The listing builds one solid part. Answer for the finished solid, in the listing's coordinates (mm). A direction names the side the tool comes from. Give positions to 0.01 mm unless a question says otherwise; leave off trailing zeros. Order: outer loops, then holes, each group sorted by start corner. A loop starts at its lowest first (then second) coordinate and runs counter-clockwise, first axis right, second up. Notation, with made-up numbers: (69.25, 3.25) - (125.25, 3.25) arc R28 ccw to (125.25, 38.25) - close; hole circle Ø8 at (83, -20.5). An arc over 180 degrees is marked (long way). Use CSV: the item, a comma, the result in double quotes.
Autodesk Inventor part; units mm, degrees
ref_plane "YZ Plane" through (0, 0, 0) normal (1, 0, 0) x (0, 1, 0)
ref_plane "XZ Plane" through (0, 0, 0) normal (0, 1, 0) x (-1, 0, 0)
ref_plane "XY Plane" through (0, 0, 0) normal (0, 0, 1) x (1, 0, 0)
sketch "Sketch1" plane through (0, 0, 0) normal (0, 0, 1) x (1, 0, 0)
  arc A0 (18.1843, -16.5324) -> (18.7618, -13.101) centre (16.0629, -14.4111) ccw
  arc A1 (18.7618, 13.101) -> (18.7618, -13.101) centre (45.75, 0) ccw
  arc A2 (18.7618, 13.101) -> (18.1843, 16.5324) centre (16.0629, 14.4111) ccw
  line L0 (11.5324, 23.1843) -> (18.1843, 16.5324)
  arc A3 (11.5324, 23.1843) -> (8.101, 23.7618) centre (9.4111, 21.0629) ccw
  arc A4 (-18.101, 23.7618) -> (8.101, 23.7618) centre (-5, 50.75) ccw
  arc A5 (-18.101, 23.7618) -> (-21.5324, 23.1843) centre (-19.4111, 21.0629) ccw
  line L1 (-28.1843, 16.5324) -> (-21.5324, 23.1843)
  arc A6 (-28.1843, 16.5324) -> (-28.7618, 13.101) centre (-26.0629, 14.4111) ccw
  arc A7 (-28.7618, -13.101) -> (-28.7618, 13.101) centre (-55.75, 0) ccw
  arc A8 (-28.7618, -13.101) -> (-28.1843, -16.5324) centre (-26.0629, -14.4111) ccw
  line L2 (-21.5324, -23.1843) -> (-28.1843, -16.5324)
  arc A9 (-21.5324, -23.1843) -> (-18.101, -23.7618) centre (-19.4111, -21.0629) ccw
  arc A10 (8.101, -23.7618) -> (-18.101, -23.7618) centre (-5, -50.75) ccw
  arc A11 (8.101, -23.7618) -> (11.5324, -23.1843) centre (9.4111, -21.0629) ccw
  line L3 (18.1843, -16.5324) -> (11.5324, -23.1843)
  circle A12 centre (10, -15) radius 4
  circle A13 centre (-20, -15) radius 4
  circle A14 centre (-20, 15) radius 4
  circle A15 centre (10, 15) radius 4
  circle A16 centre (-5, 0) radius 13
  line L4 (39.4645, -4.5) -> (34.9645, -4.5)
  line L5 (34.9645, -4.5) -> (34.9645, 4.5)
  line L6 (34.9645, 4.5) -> (39.4645, 4.5)
  line L7 (39.4645, 4.5) -> (39.4645, 10)
  line L8 (39.4645, 10) -> (31.4645, 10)
  line L9 (31.4645, 10) -> (31.4645, -10)
  line L10 (31.4645, -10) -> (39.4645, -10)
  line L11 (39.4645, -10) -> (39.4645, -4.5)
  line L12 (31.4645, -10) -> (31.4645, -17.0711)
  line L13 (31.4645, -17.0711) -> (24.4726, -24.0629)
  line L14 (31.4645, 10) -> (31.4645, 17.0711)
  line L15 (-19.4111, -24.0629) -> (24.4726, -24.0629)
  line L16 (-19.4111, 24.0629) -> (24.4726, 24.0629)
  line L17 (31.4645, 17.0711) -> (24.4726, 24.0629)
  circle A17 centre (-78.5, 0) radius 12.5
  line L18 (-19.9788, -24.0087) -> (-80.8656, -12.2741)
  line L19 (-80.8656, 12.2741) -> (-19.9788, 24.0087)
  point P0 (0, 0)
  dimension "d0" = 45
  dimension "d1" = 5
  dimension "d4" = 78.5
  dimension "d5" = 25
extrude "Extrusion1" add sketch "Sketch1" along normal blind 10 contours L3 A11 A10 A9 L2 A8 A7 A6 L1 A5 A4 A3 L0 A2 A1 A0 | A0 A1 A2 L0 A3 L16 L17 L14 L9 L12 L13 L15 A11 L3 | L15 A9 A10 A11 | L18 A17 L19 A5 L1 A6 A7 A8 L2 A9 | A3 A4 A5 L16 | A17
sketch "Sketch2" plane through (0, 0, 0) normal (0, 0, -1) x (-1, 0, 0)
  line L0 (-24.4726, -24.0629) -> (-31.4645, -17.0711)
  line L1 (19.4111, -24.0629) -> (-24.4726, -24.0629)
  arc A0 (19.4111, -24.0629) -> (19.9788, -24.0087) centre (19.4111, -21.0629) ccw
  line L2 (80.8656, -12.2741) -> (19.9788, -24.0087)
  arc A1 (80.8656, -12.2741) -> (80.8656, 12.2741) centre (78.5, 0) ccw
  line L3 (19.9788, 24.0087) -> (80.8656, 12.2741)
  arc A2 (19.9788, 24.0087) -> (19.4111, 24.0629) centre (19.4111, 21.0629) ccw
  line L4 (-24.4726, 24.0629) -> (19.4111, 24.0629)
  line L5 (-31.4645, 17.0711) -> (-24.4726, 24.0629)
  line L6 (-31.4645, -17.0711) -> (-31.4645, 17.0711)
  circle A3 centre (-10, -15) radius 4
  circle A4 centre (20, -15) radius 4
  circle A5 centre (20, 15) radius 4
  circle A6 centre (-10, 15) radius 4
  circle A7 centre (5, 0) radius 13
  line L7 (-31.4645, 17.0711) -> (-23.4645, 17.0711)
  line L8 (-23.4645, 17.0711) -> (-23.4645, -17.0711)
  line L9 (-24.4726, -24.0629) -> (-31.4645, -17.0711)
  line L10 (-23.4645, -17.0711) -> (-31.4645, -17.0711)
  line L11 (-23.4645, 17.0711) -> (-19.4726, 21.0629)
  line L12 (-19.4726, 21.0629) -> (-19.4726, 24.0629)
  line L13 (-23.4645, -17.0711) -> (-19.4726, -21.0629)
  line L14 (-19.4726, -21.0629) -> (-19.4726, -24.0629)
  line L15 (19.4111, -24.0629) -> (-24.4726, -24.0629)
  point P0 (0, 0)
  dimension "d6" = 8
  dimension "d9" = 3
extrude "Extrusion2" add sketch "Sketch2" along normal blind 29.9 contours L0 L10 L13 L14 L1 | L6 L7 L8 L10 | L5 L4 L12 L11 L7
sketch "Sketch3" plane through (23.4645, -17.0711, 0) normal (-1, 0, 0) x (0, 0, 1)
  line L0 (0, 34.1421) -> (0, 0)
  line L1 (0, 34.1421) -> (-29.9, 34.1421)
  line L2 (-29.9, 0) -> (-29.9, 34.1421)
  line L3 (0, 0) -> (-29.9, 0)
  point P0 (0, 17.0711)
  point P1 (-1.95, 25.0158)
  point P2 (-17.95, 25.0158)
  point P3 (-17.95, 10.0158)
  point P4 (-1.95, 10.0158)
  dimension "d10" = 15
  dimension "d11" = 16
  dimension "d12" = 11.95
hole "Hole1" at (23.4645, 7.9447, -1.95) at (23.4645, 7.9447, -17.95) at (23.4645, -7.0553, -17.95) at (23.4645, -7.0553, -1.95) direction (1, 0, 0) diameter 3.6 end through all counterbore diameter 6.5 counterbore depth 3.4
sketch "Sketch4" plane through (0, 0, 0) normal (0, 0, -1) x (-1, 0, 0)
  circle A0 centre (5, 0) radius 13
  circle A1 centre (-10, 15) radius 4
  circle A2 centre (20, 15) radius 4
  circle A3 centre (20, -15) radius 4
  circle A4 centre (-10, -15) radius 4
  line L0 (-19.4726, 24.0629) -> (-19.4726, 21.0629)
  line L1 (-19.4726, 21.0629) -> (-23.4645, 17.0711)
  line L2 (-23.4645, 17.0711) -> (-23.4645, 10.5447)
  line L3 (-23.4645, 10.5447) -> (-23.4645, 5.3447)
  line L4 (-23.4645, 5.3447) -> (-23.4645, -4.4553)
  line L5 (-23.4645, -4.4553) -> (-23.4645, -9.6553)
  line L6 (-23.4645, -9.6553) -> (-23.4645, -17.0711)
  line L7 (-23.4645, -17.0711) -> (-19.4726, -21.0629)
  line L8 (-19.4726, -21.0629) -> (-19.4726, -24.0629)
  line L9 (19.4111, -24.0629) -> (-19.4726, -24.0629)
  arc A5 (19.4111, -24.0629) -> (19.9788, -24.0087) centre (19.4111, -21.0629) ccw
  line L10 (80.8656, -12.2741) -> (19.9788, -24.0087)
  arc A6 (80.8656, -12.2741) -> (80.8656, 12.2741) centre (78.5, 0) ccw
  line L11 (19.9788, 24.0087) -> (80.8656, 12.2741)
  arc A7 (19.9788, 24.0087) -> (19.4111, 24.0629) centre (19.4111, 21.0629) ccw
  line L12 (-19.4726, 24.0629) -> (19.4111, 24.0629)
  line L13 (-19.4726, 21.0629) -> (-15.4807, 17.0711)
  line L14 (-15.4807, 17.0711) -> (-15.4807, -17.0711)
  line L15 (-15.4807, -17.0711) -> (-19.4726, -21.0629)
  line L16 (-23.4645, 17.0711) -> (-19.4726, 21.0629)
  point P0 (0, 0)
extrude "Extrusion3" cut sketch "Sketch4" against normal blind 2 contours L13 L14 L15 L7 L6 L5 L4 L3 L2 L1
properties part number "Corner Z Axis Carriage" material "ABS Plastic"
Item 1: The part is cut by section C-C (z = -1.95). Give the vertices of the cut face in (x, y), and give its area (3 significant figures).
Taken from the geometry:
outline,"(19.47, -24.06) - (24.47, -24.06) - (31.46, -17.07) - (31.46, -8.86) - (26.86, -8.86) - (26.86, -10.31) - (23.46, -10.31) - (23.46, -17.07) - (19.47, -21.06) - close; (19.47, 21.06) - (23.46, 17.07) - (23.46, 11.19) - (26.86, 11.19) - (26.86, 9.74) - (31.46, 9.74) - (31.46, 17.07) - (24.47, 24.06) - (19.47, 24.06) - close; (23.46, -3.81) - (26.86, -3.81) - (26.86, -5.26) - (31.46, -5.26) - (31.46, 6.14) - (26.86, 6.14) - (26.86, 4.69) - (23.46, 4.69) - close"
area,"299 mm^2"
Item 2: Find the intervals of material crossed by line 1 along Y through (x, z) = (10, 5.5); line 2 along Y through (x, z) = (25.7, -1.95); line 3 along X through (y, z) = (10.5, 1.5), in increasing order.
Taken from the geometry:
line 1,"-24.06 to -19, -11 to 11, 19 to 24.06"
line 2,"-22.84 to -10.31, -3.81 to 4.69, 11.19 to 22.84"
line 3,"-85.28 to -12.66, 2.66 to 15.48, 23.46 to 31.46"
Item 3: The mould has two halves that part along X. Classify faces 4 (the face through (-37, 0, 0)), 5 (the face through (28.017, 20.518, -10.229)), 6 (the face through (-20.521, -18.966, 4.93)), 7 (the face through (7.05, -17.7, 4.93)): +X half, -X half, draft (parallel to the pull), parting line (faces both ways), or undercut.
Taken from the geometry:
face 4,"draft"
face 5,"+X half"
face 6,"undercut"
face 7,"undercut"
Item 4: The part is cut by section B-B (y = 0). Give the vertices of the cut face in (x, z), and give its area (3 significant figures).
Taken from the geometry:
outline,"(-91, 0) - (-18, 0) - (-18, 10) - (-91, 10) - close; (8, 0) - (15.48, 0) - (15.48, 2) - (23.46, 2) - (23.46, -29.9) - (31.46, -29.9) - (31.46, 10) - (8, 10) - close"
area,"1,190 mm^2"
Item 5: The part is cut by section A-A (x = 10). Give the vertices of the cut face in (y, z).
Taken from the geometry:
outline,"(-24.06, 0) - (-19, 0) - (-19, 10) - (-24.06, 10) - close; (-11, 0) - (11, 0) - (11, 10) - (-11, 10) - close; (19, 0) - (24.06, 0) - (24.06, 10) - (19, 10) - close"
Item 6: Each of these flat-tipped pins is pushed along its axis until it touches: pin 1 (1.9 mm diameter, centred on y = -5.5, z = -2.5, fed in from -X); pin 2 (6 mm diameter, centred on x = 9.5, z = -2, fed in from +Y); pin 3 (4 mm diameter, centred on x = -41.5, z = 1, fed in from +Y); pin 4 (6.5 mm diameter, centred on x = 18.5, y = -5, fed in from -Z). Where does it stop, or does it pass through?
Taken from the geometry:
pin 1,"x = 26.86"
pin 2,"y = 24.06"
pin 3,"y = 20.25"
pin 4,"z = 0"
Item 7: The part is cut by section D-D (z = -13). Give the vertices of the cut face in (x, y), and give its area (3 significant figures).
Taken from the geometry:
outline,"(19.47, -24.06) - (24.47, -24.06) - (31.46, -17.07) - (31.46, 17.07) - (24.47, 24.06) - (19.47, 24.06) - (19.47, 21.06) - (23.46, 17.07) - (23.46, -17.07) - (19.47, -21.06) - close"
area,"376 mm^2"
Item 8: Which of the six approach directions +Z, -Z, +X, -X, +Y, -Y give full straight-line access (tool end or side, diameter ignored) to faces 1 (the face through (25.188, 7.802, -21.197)), 2 (the face through (20, 0, 2)), 3 (the face through (29.2, -8.84, -2.18))?
Taken from the geometry:
face 1,"-X"
face 2,"-Z"
face 3,"+X, -X"
